Verification items for the finished model (mm, model axes). Face numbers are marked on the shaded views. Round coordinates to 2 decimals unless told otherwise and drop trailing zeros. Loops run counter-clockwise (first coordinate to the right, second up) from the corner with the lowest first, then second, coordinate; pieces in that order, holes last. Notation, with made-up numbers: (84.5, 56.25) -> (91.5, 56.25) arc R28 ccw to (91.5, 85.25) -> close; hole circle Ø1 at (52.25, 38.5). An arc over 180 degrees is marked (long way). Write item = value, one per line. Start each with the question number.
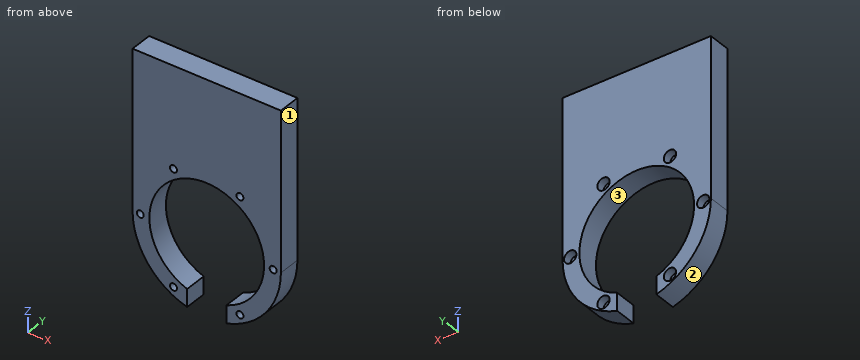
```python
from build123d import *

# Parameters (mm, degrees)
SKETCH1_R           = 26.5
BOSS_EXTRUDE1_DEPTH = 8
SKETCH2_R           = 20.5
CUT_EXTRUDE1_DEPTH  = 8
SKETCH3_W           = 14
SKETCH3_H           = 29.703096534
CUT_EXTRUDE2_DEPTH  = 15
BOSS_EXTRUDE2_START = -8
BOSS_EXTRUDE2_DEPTH = 8
SKETCH5_R           = 1.25
CUT_EXTRUDE3_DEPTH  = 8
SKETCH6_R           = 2.2
CUT_EXTRUDE4_DEPTH  = 3


with BuildPart() as part:
    # Sketch1 → Boss-Extrude1 (new body)
    with BuildSketch(Plane(origin=(0, 0, 0), x_dir=(1, 0, 0), z_dir=(0, 1, 0))):
        with Locations(Location((0, 0, 0), (0, 0, 270))):
            Circle(SKETCH1_R)
    extrude(amount=BOSS_EXTRUDE1_DEPTH)

    # Sketch2 → Cut-Extrude1 (cut)
    with BuildSketch(Plane(origin=(0, 8, 0), x_dir=(1, 0, 0), z_dir=(0, 1, 0))):
        with Locations(Location((0, 0, 0), (0, 0, 270))):
            Circle(SKETCH2_R)
    extrude(amount=-CUT_EXTRUDE1_DEPTH, mode=Mode.SUBTRACT)

    # Sketch3 → Cut-Extrude2 (cut)
    with BuildSketch(Plane(origin=(0, 8, 0), x_dir=(1, 0, 0), z_dir=(0, 1, 0))):
        with Locations((0, 12.871341831)):
            Rectangle(SKETCH3_W, SKETCH3_H)
    extrude(amount=-CUT_EXTRUDE2_DEPTH, mode=Mode.SUBTRACT)

    # Sketch4 → Boss-Extrude2 (add)
    with BuildSketch(Plane(origin=(0, 8, 0), x_dir=(1, 0, 0), z_dir=(0, 1, 0)).offset(BOSS_EXTRUDE2_START)):
        with BuildLine():
            Line((-26.5, 0), (-26.5, -56.5))
            Line((-26.5, -56.5), (26.5, -56.5))
            Line((26.5, -56.5), (26.5, 0))
            ThreePointArc((26.5, 0), (0, -26.5), (-26.5, 0))
        make_face()
    extrude(amount=BOSS_EXTRUDE2_DEPTH)

    # Sketch5 → Cut-Extrude3 (cut)
    with BuildSketch(Plane(origin=(0, 8, 0), x_dir=(1, 0, 0), z_dir=(0, 1, 0))):
        with Locations(Location((23.75, 0, 0), (0, 0, 270))):
            Circle(SKETCH5_R)
        with Locations(Location((11.875, -20.56810334, 0), (0, 0, 270))):
            Circle(SKETCH5_R)
        with Locations(Location((-11.875, -20.56810334, 0), (0, 0, 270))):
            Circle(SKETCH5_R)
        with Locations(Location((-23.75, 0, 0), (0, 0, 270))):
            Circle(SKETCH5_R)
        with Locations(Location((-11.875, 20.56810334, 0), (0, 0, 270))):
            Circle(SKETCH5_R)
        with Locations(Location((11.875, 20.56810334, 0), (0, 0, 270))):
            Circle(SKETCH5_R)
    extrude(amount=-CUT_EXTRUDE3_DEPTH, mode=Mode.SUBTRACT)

    # Sketch6 → Cut-Extrude4 (cut)
    with BuildSketch(Plane(origin=(0, 8, 0), x_dir=(1, 0, 0), z_dir=(0, 1, 0))):
        with Locations(Location((23.75, 0, 0), (0, 0, 270))):
            Circle(SKETCH6_R)
        with Locations(Location((11.875, -20.56810334, 0), (0, 0, 270))):
            Circle(SKETCH6_R)
        with Locations(Location((-11.875, -20.56810334, 0), (0, 0, 270))):
            Circle(SKETCH6_R)
        with Locations(Location((-23.75, 0, 0), (0, 0, 270))):
            Circle(SKETCH6_R)
        with Locations(Location((-11.875, 20.56810334, 0), (0, 0, 270))):
            Circle(SKETCH6_R)
        with Locations(Location((11.875, 20.56810334, 0), (0, 0, 270))):
            Circle(SKETCH6_R)
    extrude(amount=-CUT_EXTRUDE4_DEPTH, mode=Mode.SUBTRACT)


solid = part.part
```
(1) Draft check along X on the marked faces 1, 2 and 3. Enter one of: +X half, -X half, draft (parallel to the pull), parting line (faces both ways), or undercut.
(2) Section check C-C on x = -23.75. Enter the section's corners in (y, z).
(3) Section check B-B on y = 1. Enter the section's corners in (x, z) (3 decimals), then the cut area to 3 significant figures.
(4) Section check D-D on x = 0. Enter the section's corners in (y, z), then the cut area to 3 significant figures.
(5) Depth check by flat-ended pin: pin 1 Ø1.3 at (x, z) = (12.5, 21) entering from +Y; pin 2 Ø1.5 at (y, z) = (4, -4.5) entering from -X; pin 3 Ø4 at (y, z) = (4.5, -2.5) entering from +X. Enter the tip coordinate at first touch or a pass-through.
(6) Section check A-A on z = -4.5. Enter the section's corners in (x, y).
(7) Scan lines: line 1 (X direction, y = 6.05, z = 0); line 2 (Z direction, x = 22, y = 7); line 3 (X direction, y = 3.25, z = 5.5). Record each from-to range of solid material in increasing order. Write a range as [from, to].
Computed values:
q1.face_1 = +X half
q1.face_2 = -X half
q1.face_3 = undercut
q2.outline = (0, -11.76) -> (8, -11.76) -> (8, -2.2) -> (5, -2.2) -> (5, -1.25) -> (0, -1.25) -> close; (0, 1.25) -> (5, 1.25) -> (5, 2.2) -> (8, 2.2) -> (8, 56.5) -> (0, 56.5) -> close
q3.outline = (-26.5, 0) arc R26.5 ccw to (-7, -25.559) -> (-7, -19.268) arc R20.5 cw (long way) to (7, -19.268) -> (7, -25.559) arc R26.5 ccw to (26.5, 0) -> (26.5, 56.5) -> (-26.5, 56.5) -> close; hole circle Ø2.5 at (-23.75, 0); hole circle Ø2.5 at (-11.875, -20.568); hole circle Ø2.5 at (-11.875, 20.568); hole circle Ø2.5 at (11.875, -20.568); hole circle Ø2.5 at (11.875, 20.568); hole circle Ø2.5 at (23.75, 0)
q3.area = 2,660 mm²
q4.outline = (0, 20.5) -> (8, 20.5) -> (8, 56.5) -> (0, 56.5) -> close
q4.area = 288 mm²
q5.pin_1 = 5
q5.pin_2 = -26.23
q5.pin_3 = 26.5
q6.outline = (-26.12, 0) -> (-20, 0) -> (-20, 8) -> (-26.12, 8) -> close; (20, 0) -> (26.12, 0) -> (26.12, 8) -> (20, 8) -> close
q7.line_1 = [-26.5, -25.95], [-21.55, -20.5], [20.5, 21.55], [25.95, 26.5]
q7.line_2 = [-14.77, -1.33], [1.33, 56.5]
q7.line_3 = [-26.5, -19.75], [19.75, 26.5]
